Job drawing, mm, ordinate dimensions from the low corner. One solid piece. A direction names the side the tool comes from. Give positions to 0.01 mm unless a question says otherwise; leave off trailing zeros. Write each loop counter-clockwise with the first axis right and the second up, starting at its lowest first coordinate (ties: lowest second). Pieces come first, ordered by that corner, then holes. Notation, with made-up numbers: M 23,2.25 L 74,2.25 A22 ccw 74,16.25 Z; hole C -32.75,7.25 d1. An arc over 180 degrees is marked long. Use CSV: the item, a comma, the result in double quotes. Start each with the question number.
Item 1: Cut at A-A (y = 10). List the corners of the cut face in (x, z), then the cut area to 4 significant figures.
Item 2: Cut at D-D (x = 51.5). List the corners of the cut face in (y, z).
Item 3: Which spindle directions (+Z, -Z, +X, -X, +Y, -Y) get a long thin tool onto all of the face, cutting with end or side? Do the marked faces 1 and 2. Say none if no direction does.
Item 4: Drill centre lines: line 1 (Y direction, x = 1.3, z = 10); line 2 (Y direction, x = 53, z = 1.25); line 3 (Z direction, x = 1.1, y = 10). Where is each one in solid material? Low to high. Write a range as [from, to].
Item 5: Cut at B-B (z = 1.75). List the corners of the cut face in (x, y), then the cut area to 3 significant figures.
Item 6: Cut at C-C (z = 10). List the corners of the cut face in (x, y), then the cut area to 3 significant figures.
Item 7: Pin check, flat tips, straight feed: pin 1 (10 mm diameter, centred on y = 20.5, z = 9, fed in from +X); pin 2 (8 mm diameter, centred on x = 54.5, y = 16, fed in from +Z); pin 3 (5 mm diameter, centred on y = 10, z = 10, fed in from +X). Stop position of each tip, or through.
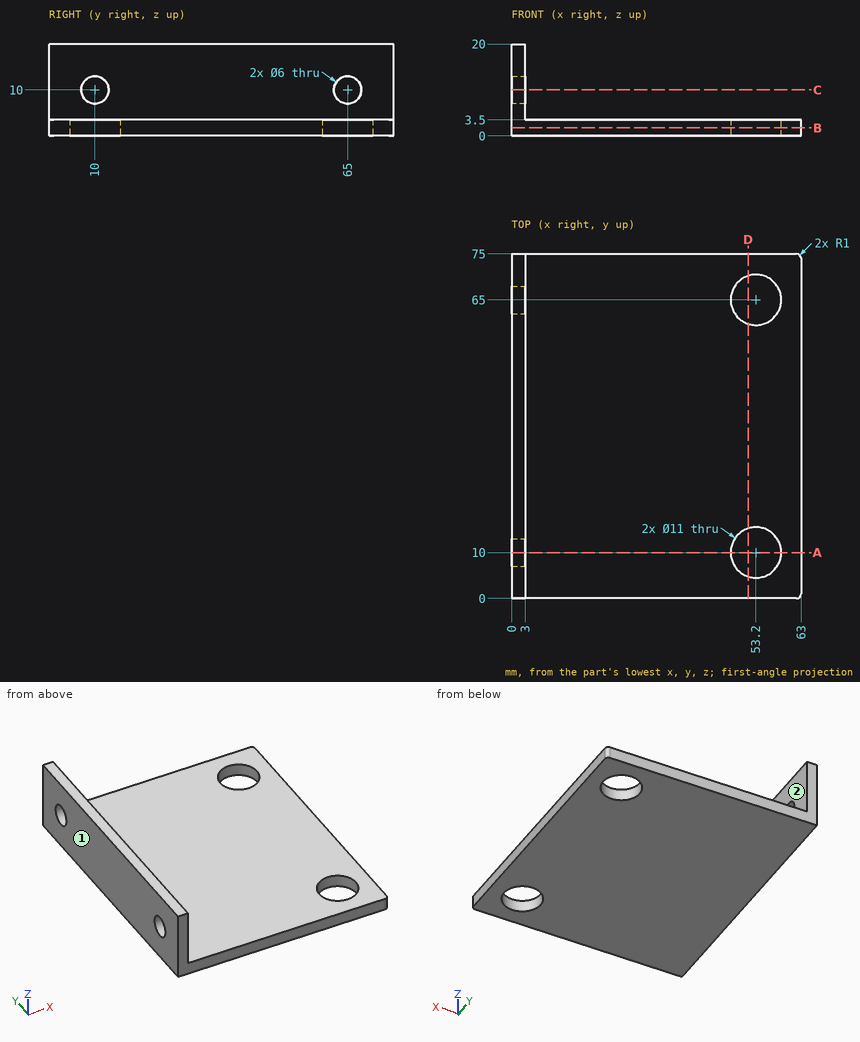
Worked answers:
1,outline,"M 0,0 L 47.7,0 L 47.7,3.5 L 3,3.5 L 3,7 L 0,7 Z; M 0,13 L 3,13 L 3,20 L 0,20 Z; M 58.7,0 L 63,0 L 63,3.5 L 58.7,3.5 Z"
1,area,"213.5 mm^2"
2,outline,"M 0,0 L 4.77,0 L 4.77,3.5 L 0,3.5 Z; M 15.23,0 L 59.77,0 L 59.77,3.5 L 15.23,3.5 Z; M 70.23,0 L 75,0 L 75,3.5 L 70.23,3.5 Z"
3,face 1,"+Z, -Z, -X, +Y, -Y"
3,face 2,"+Z, +X, +Y, -Y"
4,line 1,"y = [0, 7], [13, 62], [68, 75]"
4,line 2,"y = [0, 4.5], [15.5, 59.5], [70.5, 75]"
4,line 3,"z = [0, 7], [13, 20]"
5,outline,"M 0,0 L 62,0 A1 ccw 63,1 L 63,74 A1 ccw 62,75 L 0,75 Z; hole C 53.2,10 d11; hole C 53.2,65 d11"
5,area,"4,530 mm^2"
6,outline,"M 0,0 L 3,0 L 3,7 L 0,7 Z; M 0,13 L 3,13 L 3,62 L 0,62 Z; M 0,68 L 3,68 L 3,75 L 0,75 Z"
6,area,"189 mm^2"
7,pin 1,"stops at x = 3"
7,pin 2,"stops at z = 3.5"
7,pin 3,"passes through"
